Geometry: see drawing. Coordinates: mm, zero at the bounding-box minimum. Coordinates: 2 decimals unless noted, no trailing zeros. Order: outer loops, then holes, each group sorted by start corner. A loop starts at its lowest first (then second) coordinate and runs counter-clockwise, first axis right, second up.
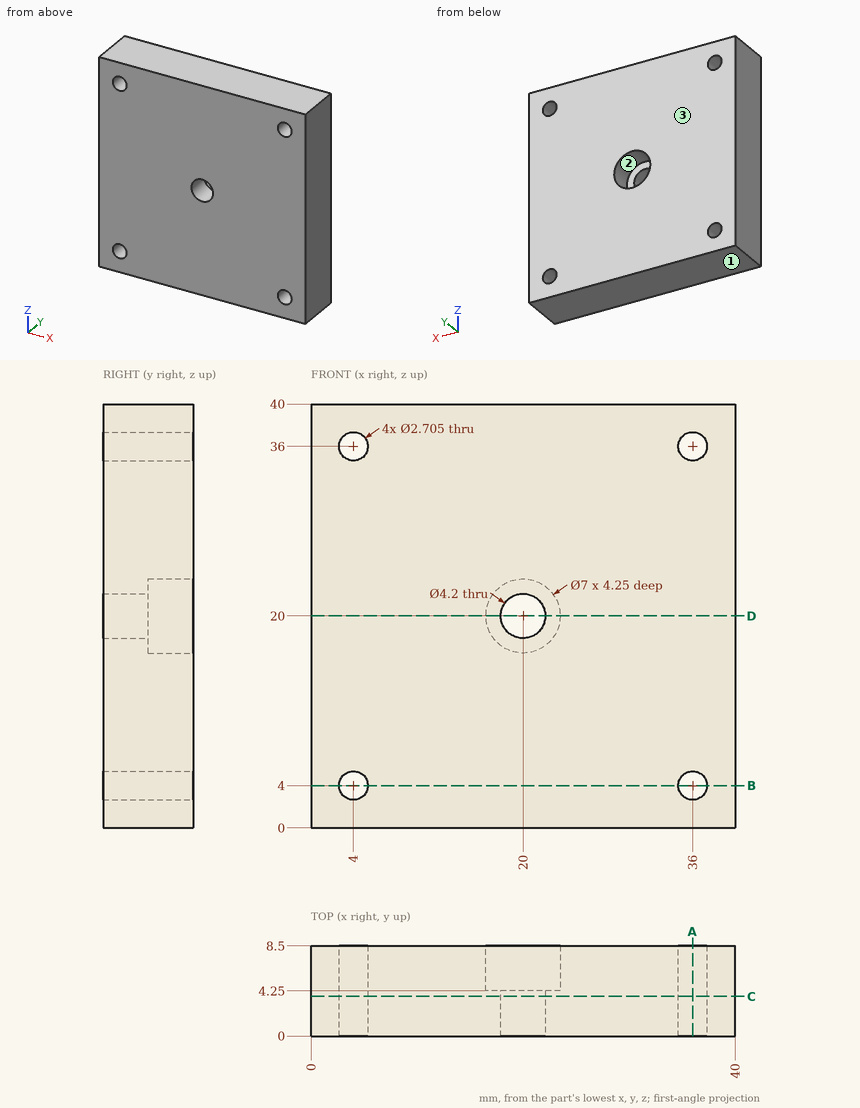
Item 1: Cut plane A-A on x = 36. Return loops of the section in (y, z), then the cut area to 3 significant figures.
Response values:
outline: (0, 0) - (8.5, 0) - (8.5, 2.65) - (0, 2.65) - close; (0, 5.35) - (8.5, 5.35) - (8.5, 34.65) - (0, 34.65) - close; (0, 37.35) - (8.5, 37.35) - (8.5, 40) - (0, 40) - close
area: 294 mm2
Item 2: Cut plane D-D on z = 20. Return loops of the section in (x, y).
Response values:
outline: (0, 0) - (17.9, 0) - (17.9, 4.25) - (16.5, 4.25) - (16.5, 8.5) - (0, 8.5) - close; (22.1, 0) - (40, 0) - (40, 8.5) - (23.5, 8.5) - (23.5, 4.25) - (22.1, 4.25) - close
Item 3: Ray query, probe 1 along Z at (x, y) = (36, 5.5); probe 2 along Z at (x, y) = (20, 5.4). Return the intervals inside material, ascending.
Response values:
probe 1: z = 0 to 2.65, 5.35 to 34.65, 37.35 to 40
probe 2: z = 0 to 16.5, 23.5 to 40
Item 4: Draft query along Z for the marked faces 1, 2 and 3. Return one class per face: pulls with the +Z half, pulls with the -Z half, needs draft (parallel to the pull), parting line crosses it, or undercut.
Response values:
face 1: pulls with the -Z half
face 2: undercut
face 3: needs draft
Item 5: Cut plane C-C on y = 3.75. Return loops of the section in (x, z) (1 decimal), then the cut area to 3 significant figures.
Response values:
outline: (0, 0) - (40, 0) - (40, 40) - (0, 40) - close; hole circle Ø2.7 at (4, 4); hole circle Ø2.7 at (4, 36); hole circle Ø4.2 at (20, 20); hole circle Ø2.7 at (36, 4); hole circle Ø2.7 at (36, 36)
area: 1,560 mm2
Item 6: Cut plane B-B on z = 4. Return loops of the section in (x, y).
Response values:
outline: (0, 0) - (2.65, 0) - (2.65, 8.5) - (0, 8.5) - close; (5.35, 0) - (34.65, 0) - (34.65, 8.5) - (5.35, 8.5) - close; (37.35, 0) - (40, 0) - (40, 8.5) - (37.35, 8.5) - close
Item 7: Pin query (flat end, axial travel): pin 1 Ø6.5 at (x, z) = (20, 20) entering from +Y. Return the tip coordinate at first contact, or that it passes through.
Response values:
pin 1: stops at y = 4.25
